from build123d import *

# Parameters (mm, degrees)
BOSS_EXTRUDE1_DEPTH    = 12.7
CUT_EXTRUDE1_DEPTH     = 31.75
M10_TAPPED_HOLE1_D     = 8.5
M10_TAPPED_HOLE1_DEPTH = 27.5
M10_TAPPED_HOLE1_TIP   = 2.553657631
M10_TAPPED_HOLE2_D     = 8.5
M10_TAPPED_HOLE2_DEPTH = 27.5
M10_TAPPED_HOLE2_TIP   = 2.553657631


with BuildPart() as part:
    # Sketch1 → Boss-Extrude1 (new, symmetric)
    with BuildSketch(Plane(origin=(0, 0, 0), x_dir=(0, 0, -1), z_dir=(1, 0, 0))):
        with BuildLine():
            Line((0, 0), (26.709237708, 0))
            ThreePointArc((26.709237708, 0), (37.074764786, 2.250146189), (45.574375763, 8.595532127))
            Line((45.574375763, 8.595532127), (158.965138054, 138.994908762))
            ThreePointArc((158.965138054, 138.994908762), (163.516110387, 146.642335221), (165.1, 155.399376635))
            Line((165.1, 155.399376635), (165.1, 184.15))
            Line((165.1, 184.15), (0, 184.15))
            Line((0, 184.15), (0, 0))
        make_face()
    extrude(amount=BOSS_EXTRUDE1_DEPTH, both=True)

    # Sketch2 → Cut-Extrude1 (cut)
    with BuildSketch(Plane(origin=(12.7, 0, 0), x_dir=(0, 0, -1), z_dir=(1, 0, 0))):
        Polygon((0, 184.15), (0, 0), (5.1, 0), (5.1, 180), (165.1, 180), (165.1, 184.15), align=None)
    extrude(amount=-CUT_EXTRUDE1_DEPTH, mode=Mode.SUBTRACT)

    # M10 Tapped Hole1
    with Locations(Plane(origin=(0, 180, 0), x_dir=(1, 0, 0), z_dir=(0, 1, 0))):
        with Locations((0, 51.100000098), (0, 101.100000098), (0, 151.100000098)):
            Hole(M10_TAPPED_HOLE1_D / 2, depth=M10_TAPPED_HOLE1_DEPTH)
            with Locations((0, 0, -(M10_TAPPED_HOLE1_DEPTH + M10_TAPPED_HOLE1_TIP / 2))):  # 118° drill point
                Cone(0, M10_TAPPED_HOLE1_D / 2, M10_TAPPED_HOLE1_TIP, mode=Mode.SUBTRACT)

    # M10 Tapped Hole2
    with Locations(Plane.XY.offset(-5.1)):
        with Locations((0, 120), (0, 88), (0, 56), (0, 24)):
            Hole(M10_TAPPED_HOLE2_D / 2, depth=M10_TAPPED_HOLE2_DEPTH)
            with Locations((0, 0, -(M10_TAPPED_HOLE2_DEPTH + M10_TAPPED_HOLE2_TIP / 2))):  # 118° drill point
                Cone(0, M10_TAPPED_HOLE2_D / 2, M10_TAPPED_HOLE2_TIP, mode=Mode.SUBTRACT)


solid = part.part
The model under review builds one solid part; all positions refer to its coordinate system, in mm. A direction names the side the tool comes from. Coordinates: 2 decimals unless noted, no trailing zeros. Loops run counter-clockwise (first coordinate to the right, second up) from the corner with the lowest first, then second, coordinate; pieces in that order, holes last.
(1) Consider section B-B, the plane x = -7.75. Give the boundary of the cut face in (y, z).
Determined:
outline: (0, -26.71) arc R25 ccw to (8.6, -45.57) - (138.99, -158.97) arc R25 ccw to (155.4, -165.1) - (180, -165.1) - (180, -5.1) - (0, -5.1) - close
(2) Draft analysis for pull direction Y (two halves, no side actions). For faces 4 (the conical face through (0.4, 150.39, -151.72)), 5 (the cylindrical face through (0.92, 166.06, -46.95)), 6 (the cylindrical face through (0.92, 51.85, -19.04)), state which applies: +Y half, -Y half, draft (parallel to the pull), parting line (faces both ways), or undercut.
Determined:
face 4: +Y half
face 5: draft
face 6: undercut
(3) Insertion check: P1, Ø5, axis at x = 0, y = 88, coming from the -Z side; P2, Ø13.5, axis at x = 0, z = -51.1, coming from the -Y side; P3, Ø4, axis at x = 2, y = 53.5, coming from the -Z side. Each pin has a flat end and moves straight along its axis. Give the tip position at first contact, or say it passes through.
Determined:
P1: stops at z = -116.8
P2: stops at y = 7.29
P3: stops at z = -86.36
(4) Consider section D-D, the plane y = 130.5. Give the boundary of the cut face in (x, z), plus the area to 3 significant figures.
Determined:
outline: (-12.7, -151.58) - (12.7, -151.58) - (12.7, -5.1) - (-12.7, -5.1) - close
area: 3,720 mm2
(5) Wall thickness on L1, parallel to Y at x = 0, z = -25; L2, parallel to Z at x = 0, y = 166; L3, parallel to X at y = 120, z = -24: over which ranges is each line inside the solid? List them lowest first.
Determined:
L1: y = 0 to 19.75, 28.25 to 51.75, 60.25 to 83.75, 92.25 to 115.75, 124.25 to 180
L2: z = -165.1 to -155.35, -146.85 to -105.35, -96.85 to -55.35, -46.85 to -5.1
L3: x = -12.7 to -4.25, 4.25 to 12.7
(6) Tool access review of faces 1 (the cylindrical face through (0.92, 166.06, -146.95)), 2 (the cylindrical face through (-2.285, 123.584, -19.043)), 3 (the cylindrical face through (0.178, 146.525, -163.472)): name each direction out of +Z, -Z, +X, -X, +Y, -Y from which nothing blocks a thin tool from reaching the whole face with its end or side.
Determined:
face 1: +Y
face 2: +Z
face 3: -Z, +X, -X, -Y
(7) Consider section A-A, the plane y = 169.5. Give the boundary of the cut face in (x, z), plus the area to 3 significant figures.
Determined:
outline: (-12.7, -165.1) - (12.7, -165.1) - (12.7, -5.1) - (-12.7, -5.1) - close; hole circle Ø8.5 at (0, -151.1); hole circle Ø8.5 at (0, -101.1); hole circle Ø8.5 at (0, -51.1)
area: 3,890 mm2
(8) Consider section C-C, the plane z = -130. Give the boundary of the cut face in (x, y) (3 decimals).
Determined:
outline: (-12.7, 105.685) - (12.7, 105.685) - (12.7, 180) - (-12.7, 180) - close
